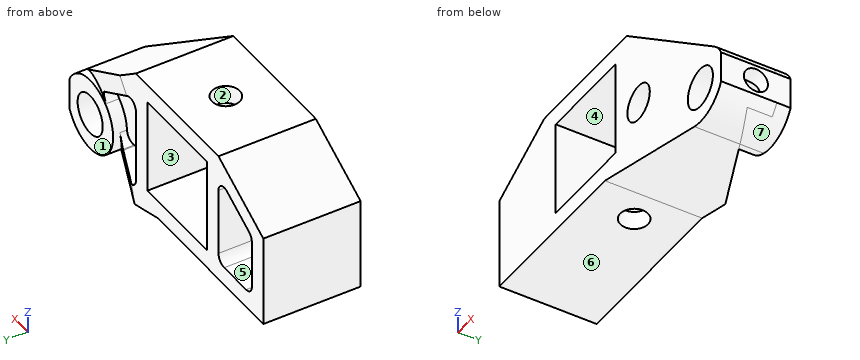
Autodesk Inventor part; units mm, degrees
ref_plane "Work Plane1" through (7.2324, 10.5, -8.3596) normal (-0.8754261, 0.4226183, 0.2345697) x (0.258819, 0, 0.9659258)
ref_plane "Work Plane2" through (8.9552, 10.5, 11.2548) normal (-0.770837, 0.258819, 0.5820851) x (-0.6026188, 0, -0.7980292)
ref_plane "YZ Plane" through (0, 0, 0) normal (1, 0, 0) x (0, 1, 0)
sketch "Sketch1" plane through (0, 0, 0) normal (0, 1, 0) x (-1, 0, 0)
  line L0 (38.625, 18.6875) -> (-38.625, 18.6875)
  line L1 (-38.625, 18.6875) -> (-38.625, -18.6875)
  line L2 (-38.625, -18.6875) -> (38.625, -18.6875)
  line L3 (38.625, -18.6875) -> (38.625, 18.6875)
  line L4 (38.625, 18.6875) -> (-38.625, -18.6875) construction
  line L5 (-38.625, 18.6875) -> (38.625, -18.6875) construction
  point P0 (0, 0)
  dimension "d0" = 77.25
  dimension "d2" = 37.375
extrude "Extrusion1" add sketch "Sketch1" along normal mid plane 21
sketch "Sketch2" plane through (0, 10.5, 0) normal (0, 1, 0) x (1, 0, 0)
  line L0 (-19, 6.0625) -> (1.75, 6.0625)
  line L1 (1.75, 6.0625) -> (1.75, -14.6875)
  line L2 (1.75, -14.6875) -> (-19, -14.6875)
  line L3 (-19, -14.6875) -> (-19, 6.0625)
  line L4 (-19, 6.0625) -> (1.75, -14.6875) construction
  line L5 (1.75, 6.0625) -> (-19, -14.6875) construction
  line L6 (-38.625, -18.6875) -> (38.625, -18.6875)
  line L7 (-38.625, 18.6875) -> (-38.625, -18.6875)
  line L8 (-38.625, 10.0625) -> (-1.8672, 10.0625)
  line L9 (-1.8672, 10.0625) -> (29.3044, 18.4149)
  arc A0 (36.196, 4.3033) -> (29.3044, 18.4149) centre (31.375, 10.6875) ccw
  line L10 (38.625, 18.6875) -> (-38.625, 18.6875)
  line L11 (36.196, 4.3033) -> (5.75, -18.6875)
  line L12 (-38.625, -9.9375) -> (-23, -18.6875)
  arc A1 (29.3044, 18.4149) -> (36.196, 4.3033) centre (31.375, 10.6875) ccw construction
  circle A2 centre (9.875, -0.3125) radius 3.9
  circle A3 centre (31.375, 10.6875) radius 4.375
  point P0 (0, 0)
  point P1 (-8.625, -4.3125)
  dimension "d5" = 20.75
  dimension "d6" = 20.75
  dimension "d7" = 4
  dimension "d8" = 19.625
  dimension "d9" = 28.75
  dimension "d10" = 16
  dimension "d11" = 70
  dimension "d12" = 44.375
  dimension "d13" = 165
  dimension "d14" = 15.625
  dimension "d15" = 8.75
  dimension "d18" = 7.8
  dimension "d19" = 18.375
  dimension "d20" = 48.5
  dimension "d21" = 8.75
extrude "Extrusion2" cut sketch "Sketch2" against normal blind 23.75 contours L12 L7 L8 L9 A0 L11 L6 keep common part
sketch "Sketch3" plane through (0, 10.5, 0) normal (0, 1, 0) x (1, 0, 0)
  line L0 (-23, 6.0625) -> (-34.625, 6.0625)
  line L1 (-34.625, 6.0625) -> (-34.625, -7.593)
  line L2 (-34.625, -7.593) -> (-23, -14.103)
  line L3 (-23, -14.103) -> (-23, 6.0625)
  line L4 (-19, 6.0625) -> (-19, -14.6875)
  line L5 (-38.625, 10.0625) -> (-1.8672, 10.0625)
  line L6 (-38.625, 10.0625) -> (-38.625, -9.9375)
  line L7 (-23, -18.6875) -> (-38.625, -9.9375)
  point P0 (0, 0)
  dimension "d22" = 4
  dimension "d23" = 4
  dimension "d24" = 4
  dimension "d25" = 4
extrude "Extrusion3" cut sketch "Sketch3" against normal blind 17
sketch "Sketch4" plane through (0, 10.5, 0) normal (0, 1, 0) x (1, 0, 0)
  line L0 (5.75, -13.6752) -> (5.75, 7.9624)
  line L1 (5.75, 7.9624) -> (23.2324, 12.6468)
  arc A0 (23.2324, 12.6468) -> (27.9136, 3.0613) centre (31.375, 10.6875) ccw
  line L2 (27.9136, 3.0613) -> (5.75, -13.6752)
  circle A1 centre (31.375, 10.6875) radius 4.375
  line L3 (-1.8672, 10.0625) -> (29.3044, 18.4149)
  line L4 (36.196, 4.3033) -> (5.75, -18.6875)
  line L5 (1.75, -14.6875) -> (1.75, 6.0625)
  point P0 (0, 0)
  dimension "d28" = 4
  dimension "d29" = 4
  dimension "d30" = 4
  dimension "d31" = 4
extrude "Extrusion4" cut sketch "Sketch4" against normal blind 9 contours L0 L1 A0 L2
fillet "Fillet1" radius 2 8 edges at (-34.625, 2, -6.0625) (-23, 2, -6.0625) (-34.625, 2, 7.593) (-23, 2, 14.103) (5.75, 6, 13.6752) (27.9136, 6, -3.0613) (5.75, 6, -7.9624) (23.2324, 6, -12.6468)
ref_plane "Work Plane1" through (7.2324, 10.5, -8.3596) normal (-0.8754261, 0.4226183, 0.2345697) x (0.258819, 0, 0.9659258)
sketch "Sketch5" plane through (7.2324, 10.5, -8.3596) normal (-0.8754261, 0.4226183, 0.2345697) x (0.258819, 0, 0.9659258)
  line L0 (-4, -3.5283) -> (-4, 10.1101)
  line L1 (0, 0) -> (0, 5.8077)
  line L2 (0, 0) -> (-4, 0)
  line L3 (-4, 0) -> (-4, 17.443)
  line L4 (-4, 17.443) -> (0, 17.443)
  line L5 (0, 17.443) -> (0, 0)
  point P0 (6.2029, -13.383)
extrude "Extrusion5" cut sketch "Sketch5" against normal blind 98.5
ref_plane "Work Plane2" through (8.9552, 10.5, 11.2548) normal (-0.770837, 0.258819, 0.5820851) x (-0.6026188, 0, -0.7980292)
sketch "Sketch6" plane through (8.9552, 10.5, 11.2548) normal (-0.770837, 0.258819, 0.5820851) x (-0.6026188, 0, -0.7980292)
  line L0 (-4, -8.053) -> (-4, 1.8213)
  line L1 (0, -5.4181) -> (0, 0)
  line L2 (0, 0) -> (-4, 0)
  line L3 (-4, 0) -> (-4, -11.4491)
  line L4 (-4, -11.4491) -> (0, -11.4491)
  line L5 (0, -11.4491) -> (0, 0)
  point P0 (14.3782, 10.2365)
extrude "Extrusion6" cut sketch "Sketch6" against normal blind 98.5
sketch "Sketch7" plane through (0, 10.5, 0) normal (0, 1, 0) x (1, 0, 0)
  line L0 (25.6612, 1.3605) -> (32.3712, 6.4274)
  arc A0 (28.6279, 14.0925) -> (32.3712, 6.4274) centre (31.375, 10.6875) ccw
  line L1 (28.6279, 14.0925) -> (20.5062, 11.9163)
  arc A1 (23.0192, 10.12) -> (20.5062, 11.9163) centre (21.0238, 9.9845) ccw
  arc A2 (23.0192, 10.12) -> (25.7898, 4.4468) centre (31.375, 10.6875) ccw
  arc A3 (25.6612, 1.3605) -> (25.7898, 4.4468) centre (24.456, 2.9565) ccw
  line L2 (35.1997, 8.5633) -> (38.625, 11.1499)
  line L3 (38.625, 11.1499) -> (38.625, 14.0694)
  arc A4 (38.625, 14.0694) -> (37.0319, 16.3444) centre (31.375, 10.6875) ccw
  line L4 (37.0319, 16.3444) -> (32.0515, 15.0099)
  arc A5 (35.1997, 8.5633) -> (32.0515, 15.0099) centre (31.375, 10.6875) ccw
  point P0 (0, 0)
extrude "Extrusion7" cut sketch "Sketch7" against normal up to surface (9 mm away)
sketch "Sketch8" plane through (0, -10.5, 0) normal (0, -1, 0) x (1, 0, 0)
  arc A0 (29.3044, -18.4149) -> (38.625, -14.0694) centre (31.375, -10.6875) ccw
  circle A1 centre (31.375, -10.6875) radius 4.375
  arc A2 (38.625, -7.3056) -> (36.196, -4.3033) centre (31.375, -10.6875) ccw
  line L0 (38.625, -14.0694) -> (38.625, -7.3056)
  line L1 (36.196, -4.3033) -> (11.3657, 14.4469)
  arc A3 (36.196, -4.3033) -> (29.3044, -18.4149) centre (31.375, -10.6875) ccw
  point P0 (0, 0)
extrude "Extrusion8" add sketch "Sketch8" against normal blind 15
fillet "Fillet2" radius 2 2 edges at (28.2566, 2.7597, -3.3203) (23.6476, 2.0377, -12.7581)
sketch "Sketch9" plane through (38.625, -10.5, -7.3056) normal (1, 0, 0) x (0, 0, -1)
  line L0 (0, 0) -> (0, 15)
  line L1 (6.7639, 0) -> (0, 0)
  line L2 (6.7639, 15) -> (6.7639, 0)
  line L3 (0, 15) -> (6.7639, 15)
  point P0 (-7.3056, 10.5)
  point P1 (3.3819, 7.5)
  point P2 (3.3819, 15)
  point P3 (6.7639, 7.5)
hole "Hole1" at (38.625, -3, -10.6875) direction (-1, 0, 0) diameter 5.2 end up to surface
sketch "Sketch10" plane through (-1.8672, 10.5, -10.0625) normal (0, 0, -1) x (-1, 0, 0)
  line L0 (-3.6172, -21) -> (17.1328, -21)
  line L1 (17.1328, 0) -> (17.1328, -21)
  line L2 (17.1328, 0) -> (-3.6172, 0)
  line L3 (-3.6172, 0) -> (-3.6172, -21)
  point P0 (-1.8672, -10.5)
  point P1 (6.7578, -10.5)
  point P2 (6.7578, 0)
  point P3 (17.1328, -10.5)
hole "Hole2" at (-8.625, 0, -10.0625) direction (0, 0, 1) diameter 6 end through all
equation "\"d6\" = d5"
equation "\"d23\" = d22"
equation "\"d24\" = d23"
equation "\"d25\" = d24"
properties part number "Y Foot Left" material "ABS Plastic"
Here's how the part is built. I have some questions about the finished solid (model axes, mm). Face numbers are marked on the shaded views. A direction names the side the tool comes from. Round coordinates to 2 decimals unless told otherwise and drop trailing zeros. Order: outer loops, then holes, each group sorted by start corner. A loop starts at its lowest first (then second) coordinate and runs counter-clockwise, first axis right, second up. Notation, with made-up numbers: (49.5, 16) -> (74.5, 16) arc R23 ccw to (74.5, 43) -> close; hole circle Ø2 at (60.25, 47). An arc over 180 degrees is marked (long way). Use a Markdown table: item, result. Add a question column.
(1) For pin 1 Ø8 at (x, y) = (14.5, 3) entering from -Z; pin 2 Ø4.5 at (y, z) = (7.5, 5) entering from +X; pin 3 Ø10 at (x, z) = (31.38, -10.69) entering from +Y, each with a flat end and sliding along its axis, tell me the tip position at first contact or that it passes through.
(2) Suppose I cut it at A-A, the plane x = -4. Please give me the cut outline in (y, z).
(3) I need wall thicknesses on line 1 along Z through (x, y) = (-3, -4); line 2 along X through (y, z) = (9, 6.5) (3 decimals); line 3 along X through (y, z) = (-1.25, 10.5). Which ranges of each line are inside material? Lowest first, please.
(4) If we mould it in two halves opening along Y, with no side actions, what happens to the marked faces 1, 2 and 3? For each: released by +Y, released by -Y, zero draft, split by the parting line, or undercut.
(5) Suppose I cut it at C-C, the plane x = 17. Please give me the cut outline in (y, z).
(6) For the marked faces 4, 5, 6 and 7, which set-ups out of +Z, -Z, +X, -X, +Y, -Y let a thin tool reach every point of the face, with its end or its side?
(7) Suppose I cut it at B-B, the plane y = 6.75. Count the separate pieces of the cut face and the enclosed holes in it, and give its area (3 significant figures).
Verdict:
| question | item | result |
|---|---|---|
| 1 | pin 1 | z = -15.52 |
| 1 | pin 2 | x = 25.66 |
| 1 | pin 3 | y = 4.5 |
| 2 | outline | (-10.5, -10.06) -> (10.5, -10.06) -> (10.5, -6.06) -> (-10.5, -6.06) -> close; (-10.5, 14.69) -> (10.5, 14.69) -> (10.5, 18.69) -> (-10.5, 18.69) -> close |
| 3 | line 1 | -10.06 to -6.06, 14.69 to 18.69 |
| 3 | line 2 | -38.625 to -34.623, -23 to -19, 1.75 to 5.75 |
| 3 | line 3 | -37.62 to -29.43, -23 to -19, 1.75 to 16.59 |
| 4 | face 1 | released by +Y |
| 4 | face 2 | undercut |
| 4 | face 3 | zero draft |
| 5 | outline | (-10.5, -15.12) -> (5.28, -15.12) -> (5.78, -10.98) -> (1.5, -10.98) -> (1.5, 5.18) -> (7.8, 5.18) -> (8.61, 10.19) -> (-10.5, 10.19) -> close |
| 6 | face 4 | +Y, -Y |
| 6 | face 5 | +Y |
| 6 | face 6 | -Z, -X, +Y, -Y |
| 6 | face 7 | -Z, +Y, -Y |
| 7 | separate pieces | 1 |
| 7 | enclosed holes | 2 |
| 7 | area | 711 mm2 |
